Input: part model. Units: mm. Frame: model coordinates. A direction names the side the tool comes from. Give positions to 0.01 mm unless a question says otherwise; leave off trailing zeros. Loops run counter-clockwise (first coordinate to the right, second up) from the corner with the lowest first, then second, coordinate; pieces in that order, holes last. Notation, with made-up numbers: (38.25, -35) - (96.25, -35) arc R12 cw to (96.25, -18) - close; hole circle Ø3 at (44.5, -27). An arc over 180 degrees is marked (long way). Answer as a JSON object with one key per item and string values.
from build123d import *

# Parameters (mm, degrees)
F2_DEPTH = 3
F1_W     = 2
F1_H     = 4
F3_DEPTH = 3


with BuildPart() as f2:
    # F0 (on Front) → F2 (new body)
    with BuildSketch(Plane.XZ):
        Polygon((4.470963, 15.720311), (-6.529037, 15.720311), (-9.589446, 9.424765), (-9.589446, 3.424765), (7.410554, 3.424765), (7.528967, 9.423597), align=None)
    extrude(amount=F2_DEPTH)

    # F1 (on Front) → F3 (cut)
    with BuildSketch(Plane.XZ):
        with Locations((4.495724, 8.424765)):
            Rectangle(F1_W, F1_H)
        with Locations((-0.999158, 10.720311)):
            Rectangle(F1_W, F1_H)
        with Locations((-6.626463, 8.424765)):
            Rectangle(F1_W, F1_H)
    extrude(amount=F3_DEPTH, mode=Mode.SUBTRACT)


solid = f2.part
Item 1: Cut plane D-D (z = 9.75). Return loops of the section in (x, y).
Geometry check:
{"outline": "(-9.43, -3) - (-7.63, -3) - (-7.63, 0) - (-9.43, 0) - close; (-5.63, -3) - (-2, -3) - (-2, 0) - (-5.63, 0) - close; (0, -3) - (3.5, -3) - (3.5, 0) - (0, 0) - close; (5.5, -3) - (7.37, -3) - (7.37, 0) - (5.5, 0) - close"}
Item 2: Mould query, pull axis Z, two halves, no side actions, for faces 3 (the face through (-9.589, -1, 6)), 4 (the face through (-5.626, -1, 8)), 5 (the face through (6.02, -1.48, 12.53)). Classes: released by +Z, released by -Z, zero draft, split by the parting line, or undercut.
Geometry check:
{"face 3": "zero draft", "face 4": "undercut", "face 5": "released by +Z"}
Item 3: Cut plane A-A (x = 3.75). Return loops of the section in (y, z).
Geometry check:
{"outline": "(-3, 3.42) - (0, 3.42) - (0, 6.42) - (-3, 6.42) - close; (-3, 10.42) - (0, 10.42) - (0, 15.72) - (-3, 15.72) - close"}
Item 4: Cut plane B-B (y = -0.45). Return loops of the section in (x, z).
Geometry check:
{"outline": "(-9.59, 3.42) - (7.41, 3.42) - (7.53, 9.42) - (4.47, 15.72) - (-6.53, 15.72) - (-9.59, 9.42) - close; hole (-7.63, 6.42) - (-5.63, 6.42) - (-5.63, 10.42) - (-7.63, 10.42) - close; hole (-2, 8.72) - (0, 8.72) - (0, 12.72) - (-2, 12.72) - close; hole (3.5, 6.42) - (5.5, 6.42) - (5.5, 10.42) - (3.5, 10.42) - close"}
Item 5: Cut plane C-C (z = 12). Return loops of the section in (x, y).
Geometry check:
{"outline": "(-8.34, -3) - (-2, -3) - (-2, 0) - (-8.34, 0) - close; (0, -3) - (6.28, -3) - (6.28, 0) - (0, 0) - close"}
Item 6: Material intervals for line 1 (Z direction, x = -1.5, y = -1.4); line 2 (Z direction, x = -6.5, y = -0.6); line 3 (X direction, y = -0.95, z = 7), sorted ascending. Write a range as [from, to].
Geometry check:
{"line 1": "z = [3.42, 8.72], [12.72, 15.72]", "line 2": "z = [3.42, 6.42], [10.42, 15.72]", "line 3": "x = [-9.59, -7.63], [-5.63, 3.5], [5.5, 7.48]"}
Item 7: Access query for faces 1 (the face through (-1, -1, 3.425)), 2 (the face through (0.001, -1, 11)). Directions: +Z, -Z, +X, -X, +Y, -Y. A direction counts if a zero-diameter tool reaches every point of the face in a straight line with its end or side. Return the directions, or none.
Geometry check:
{"face 1": "-Z, +X, -X, +Y, -Y", "face 2": "+Y, -Y"}
